Autodesk Inventor part; units mm, degrees
ref_plane "YZ Plane" through (0, 0, 0) normal (1, 0, 0) x (0, 1, 0)
ref_plane "XZ Plane" through (0, 0, 0) normal (0, 1, 0) x (-1, 0, 0)
ref_plane "XY Plane" through (0, 0, 0) normal (0, 0, 1) x (1, 0, 0)
sketch "Skizze1" plane through (0, 0, 0) normal (0, 0, 1) x (1, 0, 0)
  line L0 (-4, 0) -> (24, 0)
  line L1 (0, -1) -> (0, 6)
  line L2 (0, 2.5) -> (20, 2.5)
  line L3 (20, 2.5) -> (20, 4)
  line L4 (20, 4) -> (9, 4)
  line L5 (9, 4) -> (9, 5)
  line L6 (9, 5) -> (8, 5)
  line L7 (8, 5) -> (8, 4)
  line L8 (8, 4) -> (0, 4)
  line L9 (0, 4) -> (0, 2.5)
  point P0 (0, 0)
  dimension "d0" = 10
  dimension "d1" = 8
  dimension "d2" = 8
  dimension "d3" = 11
  dimension "d4" = 5
  dimension "d5" = 20
revolve "Umdrehung1" add sketch "Skizze1" angle 360 about axis through (-10, 0, 0) along (1, 0, 0)
fillet "Rundung1" radius 1.3 1 edges at (8, -4, 0)
properties part number "Lagerbuchse"
The listing builds one solid part. Answer for the finished solid, in the listing's coordinates (mm). A direction names the side the tool comes from. Give positions to 0.01 mm unless a question says otherwise; leave off trailing zeros. Order: outer loops, then holes, each group sorted by start corner. A loop starts at its lowest first (then second) coordinate and runs counter-clockwise, first axis right, second up. Notation, with made-up numbers: (-6, 75) - (47, 75) arc R13 ccw to (47, 81) - close; hole circle Ø6 at (70, -31). An arc over 180 degrees is marked (long way). One line per item, written item: value. Start each with the question number.
1) Given pin 1 Ø1.5 at (x, z) = (7, 3) entering from -Y; pin 2 Ø1 at (x, z) = (6, 0.5) entering from +Y, each flat-ended and moving along its own axis, determine where each tip first touches the part or whether it passes through.
2) A tool of negligible diameter and unlimited length cuts with its end or side. For faces 4 (the face through (14.423, -0.867, 3.905)), 5 (the face through (3.32, -0.867, 3.905)), 6 (the face through (20, 2, 2)), from which of +Z, -Z, +X, -X, +Y, -Y can it reach the whole face along a straight path? Write none if from no direction.
3) Find the intervals of material crossed by L1, parallel to Z at x = 5.75, y = 0; L2, parallel to Z at x = 15, y = 0.75; L3, parallel to Y at x = 6, z = -1.5, in increasing order.
4) A cutting plane is placed at C-C on x = 11.5. Give the vertices of the cut face in (y, z), then the cut area to 3 significant figures.
5) The mould has two halves that part along Z. Classify faces 1 (the face through (8.49, -1.08, 4.88)), 2 (the face through (0, 2, 2)), 3 (the face through (10.14, -0.54, -2.44)): released by +Z, released by -Z, zero draft, split by the parting line, or undercut.
6) A cutting plane is placed at A-A on z = 0. Give the vertices of the cut face in (x, y).
Answer sheet:
1. pin 1: stops at y = -3.5
1. pin 2: stops at y = 4
2. face 4: +X
2. face 5: -X
2. face 6: +Z, -Z, +X, +Y, -Y
3. L1: z = -4 to -2.5, 2.5 to 4
3. L2: z = -3.93 to -2.38, 2.38 to 3.93
3. L3: y = -3.71 to -2, 2 to 3.71
4. outline: circle Ø8 at (0, 0); hole circle Ø5 at (0, 0)
4. area: 30.6 mm2
5. face 1: split by the parting line
5. face 2: zero draft
5. face 3: undercut
6. outline: (0, -4) - (6.74, -4) arc R1.3 cw to (8, -5) - (9, -5) - (9, -4) - (20, -4) - (20, -2.5) - (0, -2.5) - close; (0, 2.5) - (20, 2.5) - (20, 4) - (9, 4) - (9, 5) - (8, 5) arc R1.3 cw to (6.74, 4) - (0, 4) - close
